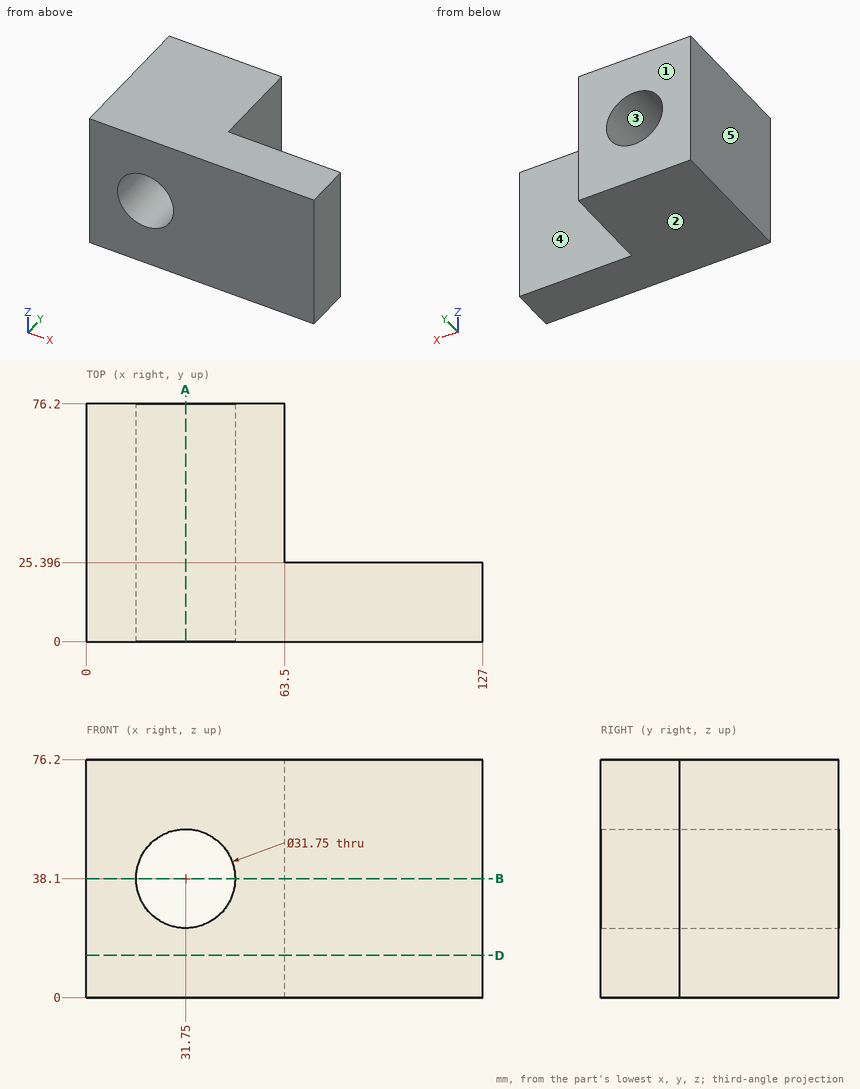
Source: three-view drawing plus pictorial views. Frame: mm from the lowest corner of the part. A direction names the side the tool comes from. Give positions to 0.01 mm unless a question says otherwise; leave off trailing zeros. Order: outer loops, then holes, each group sorted by start corner. A loop starts at its lowest first (then second) coordinate and runs counter-clockwise, first axis right, second up. Notation, with made-up numbers: M 12.25,58.25 L 43.25,58.25 A27 cw 43.25,94.25 Z; hole C 3,60 d10. An arc over 180 degrees is marked long. Return JSON: item names as keys, results as strings.
1) Section query A-A on x = 31.75. Output: boundary loops of the cut face in (y, z) (1 decimal), and give its area (3 significant figures).
Taken from the geometry:
{"outline": "M 0,0 L 76.2,0 L 76.2,22.2 L 0,22.2 Z; M 0,54 L 76.2,54 L 76.2,76.2 L 0,76.2 Z", "area": "3,390 mm2"}
2) Section query B-B on z = 38.1. Output: boundary loops of the cut face in (x, y) (1 decimal).
Taken from the geometry:
{"outline": "M 0,0 L 15.9,0 L 15.9,76.2 L 0,76.2 Z; M 47.6,0 L 127,0 L 127,25.4 L 63.5,25.4 L 63.5,76.2 L 47.6,76.2 Z"}
3) Contact query for flat-ended pins moving along their axis: pin 1 (2 mm diameter, centred on x = 70.5, z = 51, fed in from -Y); pin 2 (3 mm diameter, centred on y = 50.5, z = 18.5, fed in from +X). Output: stop coordinate, or through.
Taken from the geometry:
{"pin 1": "stops at y = 0", "pin 2": "stops at x = 63.5"}
4) Mould query, pull axis Z, two halves, no side actions, for the marked faces 1, 2 and 3. Classes: released by +Z, released by -Z, zero draft, split by the parting line, or undercut.
Taken from the geometry:
{"face 1": "zero draft", "face 2": "released by -Z", "face 3": "undercut"}
5) Access query for the marked faces 4 and 5. Directions: +Z, -Z, +X, -X, +Y, -Y. A direction counts if a zero-diameter tool reaches every point of the face in a straight line with its end or side. Return the directions, or none.
Taken from the geometry:
{"face 4": "+Z, -Z, +X, +Y", "face 5": "+Z, -Z, -X, +Y, -Y"}
6) Line query: L1, parallel to X at y = 48, z = 38.1 (1 decimal); L2, parallel to Z at x = 31.75, y = 55 (1 decimal); L3, parallel to Y at x = 112.5, z = 60 (1 decimal). Output: solid intervals per line, ascending. Write a range as [from, to].
Taken from the geometry:
{"L1": "x = [0, 15.9], [47.6, 63.5]", "L2": "z = [0, 22.2], [54, 76.2]", "L3": "y = [0, 25.4]"}
7) Section query D-D on z = 13.5. Output: boundary loops of the cut face in (x, y) (1 decimal), and give its area (3 significant figures).
Taken from the geometry:
{"outline": "M 0,0 L 127,0 L 127,25.4 L 63.5,25.4 L 63.5,76.2 L 0,76.2 Z", "area": "6,450 mm2"}
